from build123d import *

# Parameters (mm, degrees)
BOX239_W               = 25
BOX239_H               = 10
BOX239_DEPTH           = 10
BOX239_PLACEMENT_ANGLE = 10
BOX236_W               = 25
BOX236_H               = 10
BOX236_DEPTH           = 10
CYLINDER312_R          = 9
CYLINDER312_DEPTH      = 17
CYLINDER311_R          = 9
CYLINDER311_DEPTH      = 24
CYLINDER315_R          = 3
CYLINDER315_DEPTH      = 10
BOX234_W               = 21
BOX234_H               = 7
BOX234_DEPTH           = 3.5
CYLINDER317_R          = 1.25
CYLINDER317_DEPTH      = 10
CYLINDER318_R          = 6
CYLINDER318_DEPTH      = 10
CYLINDER313_R          = 2
CYLINDER313_DEPTH      = 10
BOX230_W               = 20.75
BOX230_H               = 9.25
BOX230_DEPTH           = 10
CYLINDER316_R          = 4
CYLINDER316_DEPTH      = 4
BOX233_W               = 12
BOX233_H               = 4
BOX233_DEPTH           = 8
CYLINDER310_R          = 1.6
CYLINDER310_DEPTH      = 10
CYLINDER309_R          = 1.6
CYLINDER309_DEPTH      = 10
BOX231_W               = 26
BOX231_H               = 15
BOX231_DEPTH           = 2
FILLET122_R            = 3


with BuildPart() as obj1:
    # Box239 → Box239 (new body)
    with BuildSketch(Plane.XY):
        with Locations((12.5, 5)):
            Rectangle(BOX239_W, BOX239_H)
    extrude(amount=BOX239_DEPTH)


with BuildPart() as obj1_1:
    # Box239 placement: moved
    add(obj1.part.moved(Location((10.031417, -8.25, 26.431635))).rotate(Axis((10.031417, -8.25, 26.431635), (0, 1, 0)), BOX239_PLACEMENT_ANGLE))


with BuildPart() as obj2:
    # Box236 → Box236 (new body)
    with BuildSketch(Plane(origin=(7.75, -8.25, 42), x_dir=(1, 0, 0), z_dir=(0, 0, 1))):
        with Locations((12.5, 5)):
            Rectangle(BOX236_W, BOX236_H)
    extrude(amount=BOX236_DEPTH)


with BuildPart() as zylinder314:
    # Cylinder312 → Cylinder312 (new body)
    with BuildSketch(Plane(origin=(16, 3.363861, 32.453751), x_dir=(-1, 0, 0), z_dir=(0, -1, 0))):
        Circle(CYLINDER312_R)
    extrude(amount=CYLINDER312_DEPTH)


with BuildPart() as fusion210:
    # Cylinder311 → Cylinder311 (new body)
    with BuildSketch(Plane(origin=(16.5, -14.136139, 32.703751), x_dir=(0, -1, 0), z_dir=(1, 0, 0))):
        Circle(CYLINDER311_R)
    extrude(amount=CYLINDER311_DEPTH)

    # Fusion210: union Zylinder314
    add(zylinder314.part)


with BuildPart() as zylinder317:
    # Cylinder315 → Cylinder315 (new body)
    with BuildSketch(Plane(origin=(38.25, 5.75, 36.25), x_dir=(1, 0, 0), z_dir=(0, -1, 0))):
        Circle(CYLINDER315_R)
    extrude(amount=CYLINDER315_DEPTH)


with BuildPart() as obj3:
    # Box234 → Box234 (new body)
    with BuildSketch(Plane(origin=(22.5, -4.25, 34.5), x_dir=(1, 0, 0), z_dir=(0, 0, 1))):
        with Locations((10.5, 3.5)):
            Rectangle(BOX234_W, BOX234_H)
    extrude(amount=BOX234_DEPTH)


with BuildPart() as zylinder319:
    # Cylinder317 → Cylinder317 (new body)
    with BuildSketch(Plane(origin=(38.25, 3.25, 36.25), x_dir=(1, 0, 0), z_dir=(0, -1, 0))):
        Circle(CYLINDER317_R)
    extrude(amount=CYLINDER317_DEPTH)


with BuildPart() as zylinder320:
    # Cylinder318 → Cylinder318 (new body)
    with BuildSketch(Plane(origin=(38.25, -0.5, 46.25), x_dir=(1, 0, 0), z_dir=(0, -1, 0))):
        Circle(CYLINDER318_R)
    extrude(amount=CYLINDER318_DEPTH)


with BuildPart() as fusion212:
    # Cylinder313 → Cylinder313 (new body)
    with BuildSketch(Plane(origin=(38.25, -5, 36.25), x_dir=(1, 0, 0), z_dir=(0, -1, 0))):
        Circle(CYLINDER313_R)
    extrude(amount=CYLINDER313_DEPTH)

    # Fusion212: union Zylinder317, obj3, Zylinder319, Zylinder320
    add(zylinder317.part)
    add(obj3.part)
    add(zylinder319.part)
    add(zylinder320.part)


with BuildPart() as obj4:
    # Box230 → Box230 (new body)
    with BuildSketch(Plane(origin=(17.5, -10.25, 32.25), x_dir=(1, 0, 0), z_dir=(0, 0, 1))):
        with Locations((10.375, 4.625)):
            Rectangle(BOX230_W, BOX230_H)
    extrude(amount=BOX230_DEPTH)


with BuildPart() as zylinder318:
    # Cylinder316 → Cylinder316 (new body)
    with BuildSketch(Plane(origin=(38.25, -1, 36.25), x_dir=(1, 0, 0), z_dir=(0, -1, 0))):
        Circle(CYLINDER316_R)
    extrude(amount=CYLINDER316_DEPTH)


with BuildPart() as cut146:
    # Box233 → Box233 (new body)
    with BuildSketch(Plane(origin=(26.25, -5, 32.25), x_dir=(1, 0, 0), z_dir=(0, 0, 1))):
        with Locations((6, 2)):
            Rectangle(BOX233_W, BOX233_H)
    extrude(amount=BOX233_DEPTH)

    # Fusion211: union obj4, Zylinder318
    add(obj4.part)
    add(zylinder318.part)

    # Cut145: cut Fusion212
    add(fusion212.part, mode=Mode.SUBTRACT)

    # Cut146: cut Fusion210
    add(fusion210.part, mode=Mode.SUBTRACT)


with BuildPart() as zylinder312:
    # Cylinder310 → Cylinder310 (new body)
    with BuildSketch(Plane(origin=(35, -13.75, 33.25), x_dir=(1, 0, 0), z_dir=(0, 0, 1))):
        Circle(CYLINDER310_R)
    extrude(amount=CYLINDER310_DEPTH)


with BuildPart() as fusion209:
    # Cylinder309 → Cylinder309 (new body)
    with BuildSketch(Plane(origin=(14, -13.75, 33.25), x_dir=(1, 0, 0), z_dir=(0, 0, 1))):
        Circle(CYLINDER309_R)
    extrude(amount=CYLINDER309_DEPTH)

    # Fusion209: union Zylinder312
    add(zylinder312.part)


with BuildPart() as fusion209_1:
    # Fusion209 placement: moved
    add(fusion209.part.moved(Location((0.5, 0, 5))))


with BuildPart() as cut149:
    # Box231 → Box231 (new body)
    with BuildSketch(Plane(origin=(12, -16, 41.5), x_dir=(1, 0, 0), z_dir=(0, 0, 1))):
        with Locations((13, 7.5)):
            Rectangle(BOX231_W, BOX231_H)
    extrude(amount=BOX231_DEPTH)

    # Cut144: cut Fusion209
    add(fusion209_1.part, mode=Mode.SUBTRACT)


with BuildPart() as cut149_1:
    # Cut144 placement: moved
    add(cut149.part.moved(Location((0, 1.75, 0))))

    # Fillet122
    fillet122_edges = [cut149_1.edges().sort_by_distance(p)[0] for p in [
        (12, -14.25, 42.5),
        (38, -14.25, 42.5),
    ]]
    fillet(fillet122_edges, radius=FILLET122_R)


with BuildPart() as cut149_2:
    # Fillet122 placement: moved
    add(cut149_1.part.moved(Location((-4.75, 0, 0))))

    # Fusion213: union Cut146
    add(cut146.part)

    # Cut147: cut obj2
    add(obj2.part, mode=Mode.SUBTRACT)

    # Cut149: cut obj1
    add(obj1_1.part, mode=Mode.SUBTRACT)


solid = cut149_2.part
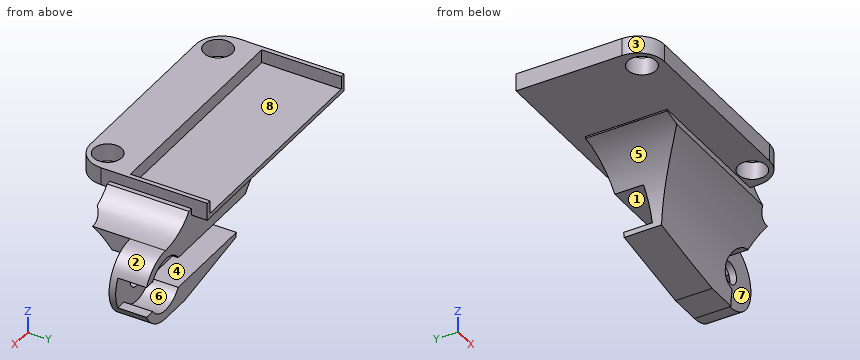
Input: part model. Units: mm. Frame: model coordinates. Face numbers are marked on the shaded views. A direction names the side the tool comes from. Round coordinates to 2 decimals unless told otherwise and drop trailing zeros. Loops run counter-clockwise (first coordinate to the right, second up) from the corner with the lowest first, then second, coordinate; pieces in that order, holes last. Notation, with made-up numbers: (-31.5, -38) -> (7.5, -38) arc R36 cw to (7.5, -2) -> close; hole circle Ø10 at (62.25, 3). An arc over 180 degrees is marked (long way). Answer as a JSON object with one key per item and string values. Group by question number.
1) Pin query (flat end, axial travel): pin 1 (1.6 mm diameter, centred on x = 28.5, y = -3, fed in from -Z); pin 2 (2 mm diameter, centred on y = -7, z = 39, fed in from +X); pin 3 (0.8 mm diameter, centred on y = -4, z = 43, fed in from +X). Return the tip coordinate at first contact, or that it passes through.
2) Section query A-A on y = -2.25. Output: boundary loops of the cut face in (x, z).
3) Reachability of the marked faces 4, 5, 6, 7 and 8 from +Z, -Z, +X, -X, +Y, -Y: full face, straight path, thin tool, end or side. Return the list, or none.
4) Section query C-C on z = 36.25. Output: boundary loops of the cut face in (x, y), plus the area to 3 significant figures.
5) Draft query along Z for the marked faces 1, 2 and 3. Return one class per face: +Z half, -Z half, draft (parallel to the pull), parting line (faces both ways), or undercut.
6) Section query D-D on y = -12. Output: boundary loops of the cut face in (x, z), plus the area to 3 significant figures.
7) Section query B-B on x = 9.75. Output: boundary loops of the cut face in (y, z), plus the area to 3 significant figures.
8) Ray query, L1, parallel to Z at x = 38.25, y = -4.5; L2, parallel to Y at x = 30.75, z = 42.8; L3, parallel to X at y = -12, z = 42.2. Return the intervals inside material, ascending.
Reply:
{
 "1": {"pin 1": "stops at z = 33.19", "pin 2": "stops at x = 38.25", "pin 3": "stops at x = 33.25"},
 "2": {"outline": "(7.25, 41.5) -> (17.5, 41.5) -> (17.5, 41.33) arc R9 cw to (23.09, 38) -> (35.81, 38) arc R3 cw to (40.69, 38) -> (41.85, 38) arc R4 ccw to (38.25, 40.25) arc R6 cw to (33.78, 42.25) -> (33.25, 42.25) -> (33.25, 43.5) -> (32.75, 43.5) -> (32.75, 42) -> (7.75, 42) -> (7.75, 43.5) -> (7.25, 43.5) -> close; (24.76, 34.5) arc R9 cw to (24.87, 33.97) -> (34.62, 32.25) -> (38.25, 32.25) arc R4 ccw to (41.85, 34.5) -> (40.69, 34.5) arc R3 cw to (35.81, 34.5) -> close"},
 "3": {"face 4": "+X, -X, +Y", "face 5": "-Z, -X, +Y, -Y", "face 6": "+Y", "face 7": "+X, -Y", "face 8": "+Z, +Y"},
 "4": {"outline": "(24.16, -5.86) -> (36.25, -5.86) -> (36.25, -5) -> (37, -5) -> (37, -4.25) -> (24.16, -4.25) -> close; (39.5, -5) -> (42.25, -5) -> (42.25, -4.25) -> (39.5, -4.25) -> close", "area": "22.1 mm2"},
 "5": {"face 1": "undercut", "face 2": "parting line", "face 3": "draft"},
 "6": {"outline": "(7.35, 41.5) -> (8.15, 41.5) -> (8.15, 43.5) -> (7.35, 43.5) -> close; (11.35, 41.5) -> (29.15, 41.5) -> (29.15, 43.5) -> (11.35, 43.5) -> close; (32.35, 41.5) -> (33.15, 41.5) -> (33.15, 43.5) -> (32.35, 43.5) -> close", "area": "38.8 mm2"},
 "7": {"outline": "(-14.21, 41.5) -> (-13.6, 41.5) -> (-13.6, 43.5) -> (-14.21, 43.5) -> close; (-10.4, 41.5) -> (0.75, 41.5) -> (0.75, 42) -> (-8.25, 42) -> (-8.25, 43.5) -> (-10.4, 43.5) -> close", "area": "10.0 mm2"},
 "8": {"L1": "z = 32.25 to 35, 37.5 to 40.25", "L2": "y = -14.21 to -13.6, -10.4 to -8.25", "L3": "x = 7.35 to 8.15, 11.35 to 29.15, 32.35 to 33.15"}
}
